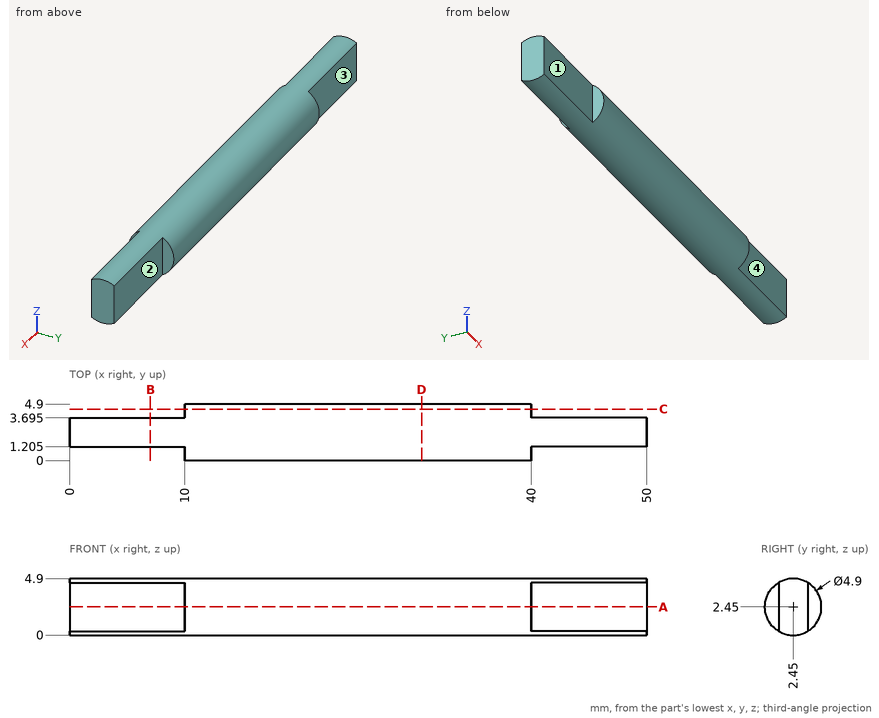
Drawing for the job (mm, zero at the part's lowest x, y, z). A direction names the side the tool comes from. Coordinates: 2 decimals unless noted, no trailing zeros. Order: outer loops, then holes, each group sorted by start corner. A loop starts at its lowest first (then second) coordinate and runs counter-clockwise, first axis right, second up. Notation, with made-up numbers: (-30, 73) - (-16, 73) arc R20 cw to (-16, 111) - close; hole circle Ø5 at (89, 58). An arc over 180 degrees is marked (long way). Use a Markdown table: item, result. Add a question column.
(1) Saw through at A-A (z = 2.45). Give the cut face in (x, y) (3 decimals).
(2) Saw through at C-C (y = 4.45). Give the cut face in (x, z), then the cut area to 3 significant figures.
(3) Flat gauge pins, fed straight in: pin 1 (1.3 mm diameter, centred on y = 4.5, z = 1.5, fed in from +X); pin 2 (0.6 mm diameter, centred on y = 0.5, z = 2, fed in from -X); pin 3 (2 mm diameter, centred on x = 46, z = 3, fed in from -Y) (3 decimals). Where does each tip first touch, or does it go through?
(4) Drill centre lines: line 1 along X through (y, z) = (0.95, 2.95); line 2 along Y through (x, z) = (42.5, 2.65) (3 decimals); line 3 along Z through (x, y) = (29.5, 1.45). Where is each one in solid material? Low to high. Write a range as [from, to].
(5) Saw through at D-D (x = 30.5). Give the cut face in (y, z), then the cut area to 3 significant figures.
(6) Saw through at B-B (x = 7). Give the cut face in (y, z) (3 decimals).
(7) Which spindle directions (+Z, -Z, +X, -X, +Y, -Y) get a long thin tool onto all of the face, cutting with end or side? Do the marked faces 1, 2, 3 and 4. Say none if no direction does.
Solved:
| question | item | result |
|---|---|---|
| 1 | outline | (0, 1.205) - (10, 1.205) - (10, 0) - (40, 0) - (40, 1.205) - (50, 1.205) - (50, 3.695) - (40, 3.695) - (40, 4.9) - (10, 4.9) - (10, 3.695) - (0, 3.695) - close |
| 2 | outline | (10, 1.03) - (40, 1.03) - (40, 3.87) - (10, 3.87) - close |
| 2 | area | 84.9 mm² |
| 3 | pin 1 | stops at x = 40 |
| 3 | pin 2 | stops at x = 10 |
| 3 | pin 3 | stops at y = 1.205 |
| 4 | line 1 | x = [10, 40] |
| 4 | line 2 | y = [1.205, 3.695] |
| 4 | line 3 | z = [0.21, 4.69] |
| 5 | outline | circle Ø4.9 at (2.45, 2.45) |
| 5 | area | 18.9 mm² |
| 6 | outline | (1.205, 0.34) arc R2.45 ccw to (3.695, 0.34) - (3.695, 4.56) arc R2.45 ccw to (1.205, 4.56) - close |
| 7 | face 1 | +Z, -Z, -X, -Y |
| 7 | face 2 | +Z, -Z, +X, +Y |
| 7 | face 3 | +Z, -Z, -X, +Y |
| 7 | face 4 | +Z, -Z, +X, -Y |
